Here's the drawing with two shaded views (mm, measured from the low corner). I have some questions. A direction names the side the tool comes from. Give positions to 0.01 mm unless a question says otherwise; leave off trailing zeros. Write each loop counter-clockwise with the first axis right and the second up, starting at its lowest first coordinate (ties: lowest second). Pieces come first, ordered by that corner, then holes. Notation, with made-up numbers: (16, 19) -> (60, 19) arc R18 cw to (60, 28) -> close; hole circle Ø3 at (75, 4). An arc over 180 degrees is marked (long way). One line per question, with ' | ' between items.
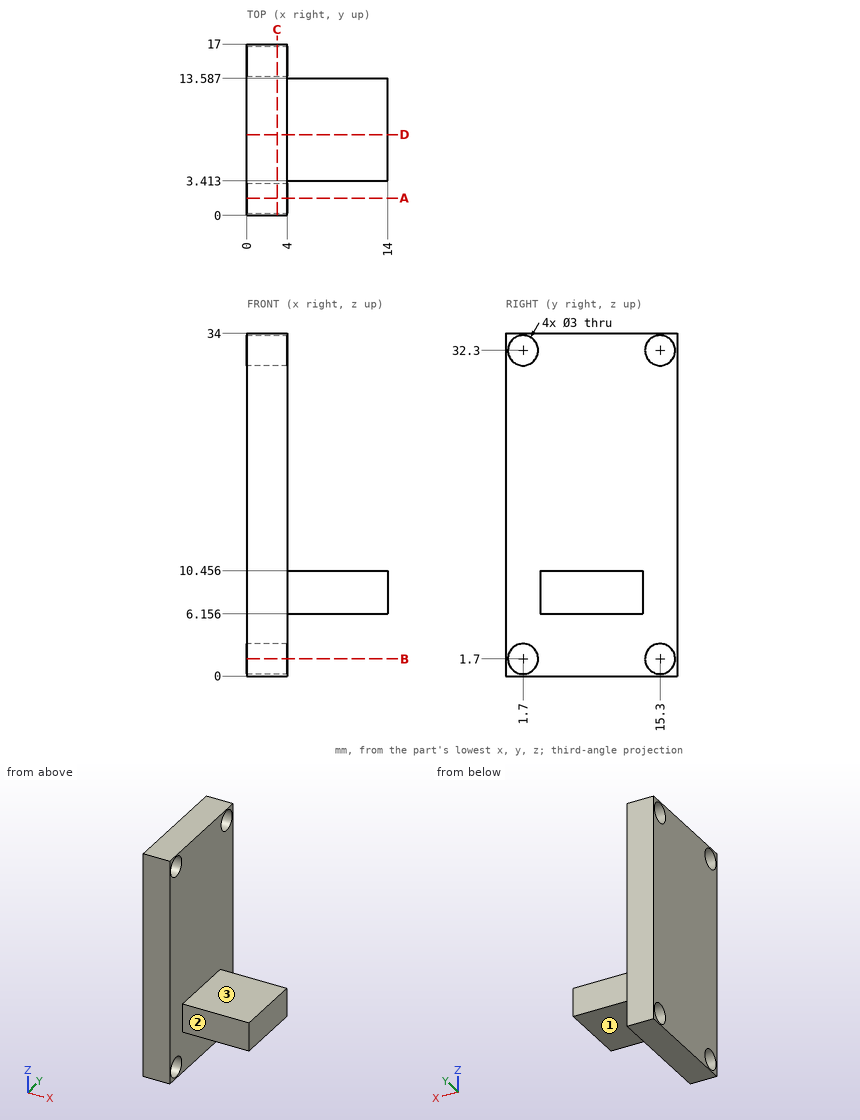
Q1. Imagine slicing it at D-D on y = 8. Please give me the cut outline in (x, z), and give its area (3 significant figures).
Answer below:
outline: (0, 0) -> (4, 0) -> (4, 6.16) -> (14, 6.16) -> (14, 10.46) -> (4, 10.46) -> (4, 34) -> (0, 34) -> close | area: 179 mm^2
Q2. Imagine slicing it at A-A on y = 1.7. Please give me the cut outline in (x, z), and give its area (3 significant figures).
Answer below:
outline: (0, 0) -> (4, 0) -> (4, 0.2) -> (0, 0.2) -> close; (0, 3.2) -> (4, 3.2) -> (4, 30.8) -> (0, 30.8) -> close; (0, 33.8) -> (4, 33.8) -> (4, 34) -> (0, 34) -> close | area: 112 mm^2
Q3. Imagine slicing it at B-B on z = 1.7. Please give me the cut outline in (x, y), and give its area (3 significant figures).
Answer below:
outline: (0, 0) -> (4, 0) -> (4, 0.2) -> (0, 0.2) -> close; (0, 3.2) -> (4, 3.2) -> (4, 13.8) -> (0, 13.8) -> close; (0, 16.8) -> (4, 16.8) -> (4, 17) -> (0, 17) -> close | area: 44.0 mm^2
Q4. Imagine slicing it at C-C on x = 3. Please give me the cut outline in (y, z), and give its area (3 significant figures).
Answer below:
outline: (0, 0) -> (17, 0) -> (17, 34) -> (0, 34) -> close; hole circle Ø3 at (1.7, 1.7); hole circle Ø3 at (1.7, 32.3); hole circle Ø3 at (15.3, 1.7); hole circle Ø3 at (15.3, 32.3) | area: 550 mm^2
Q5. Will these pins go through, and if not, where does the flat tip stop? pin 1 (2 mm diameter, centred on x = 8.5, y = 12, fed in from +Z); pin 2 (8.5 mm diameter, centred on y = 11, z = 25, fed in from +X); pin 3 (1.8 mm diameter, centred on y = 15.3, z = 1.7, fed in from -X); pin 4 (3.5 mm diameter, centred on x = 8.5, z = 9.5, fed in from +Y).
Answer below:
pin 1: stops at z = 10.46 | pin 2: stops at x = 4 | pin 3: passes through | pin 4: stops at y = 13.59
Q6. If I drill on line 1 along Y through (x, z) = (1.6, 32.3); line 2 along X through (y, z) = (10.5, 19); line 3 along Z through (x, y) = (10, 6.5), over which ranges is the centre line in solid material (lowest first)?
Answer below:
line 1: y = 0 to 0.2, 3.2 to 13.8, 16.8 to 17 | line 2: x = 0 to 4 | line 3: z = 6.16 to 10.46
Q7. On a 3-axis mill with a long thin cutter (end or side, diameter ignored), from which of +Z, -Z, +X, -X, +Y, -Y can I reach the whole of each face in a straight line? I mean the marked faces 1, 2 and 3. Say none if no direction works.
Answer below:
face 1: -Z, +X, +Y, -Y | face 2: +Z, -Z, +X, -Y | face 3: +Z, +X, +Y, -Y
